Here's the drawing with two shaded views (mm, measured from the low corner). I have some questions. Coordinates: 2 decimals unless noted, no trailing zeros. Write each loop counter-clockwise with the first axis right and the second up, starting at its lowest first coordinate (ties: lowest second). Pieces come first, ordered by that corner, then holes. Notation, with made-up numbers: M 71.25,67.5 L 113.25,67.5 A24 ccw 113.25,99.5 Z; hole C -15.5,-20 d1. An arc over 180 degrees is marked long. Use one line per item in the form item = value. Start each with the question number.
1. I want a section at A-A, the plane y = 2.25. List the corners of the cut face in (x, z) for me.
2. I want a section at B-B, the plane y = 5.25. List the corners of the cut face in (x, z) for me.
3. I'm going to push a flat-ended pin straight in: pin 1 Ø2 at (x, y) = (2, 1.5) entering from +Z. Where does the tip first touch, or does it pass through?
4. Thinking about a two-plate mould opening in X: for the marked faces 1, 2 and 3, which applies, released by +X, released by -X, zero draft, split by the parting line, or undercut?
5. Please list where these lines run through material, in increasing order: line 1 along X through (y, z) = (4.5, 2.05); line 2 along Z through (x, y) = (1.5, 4.5); line 3 along Y through (x, z) = (2.8, 1.5). Write a range as [from, to].
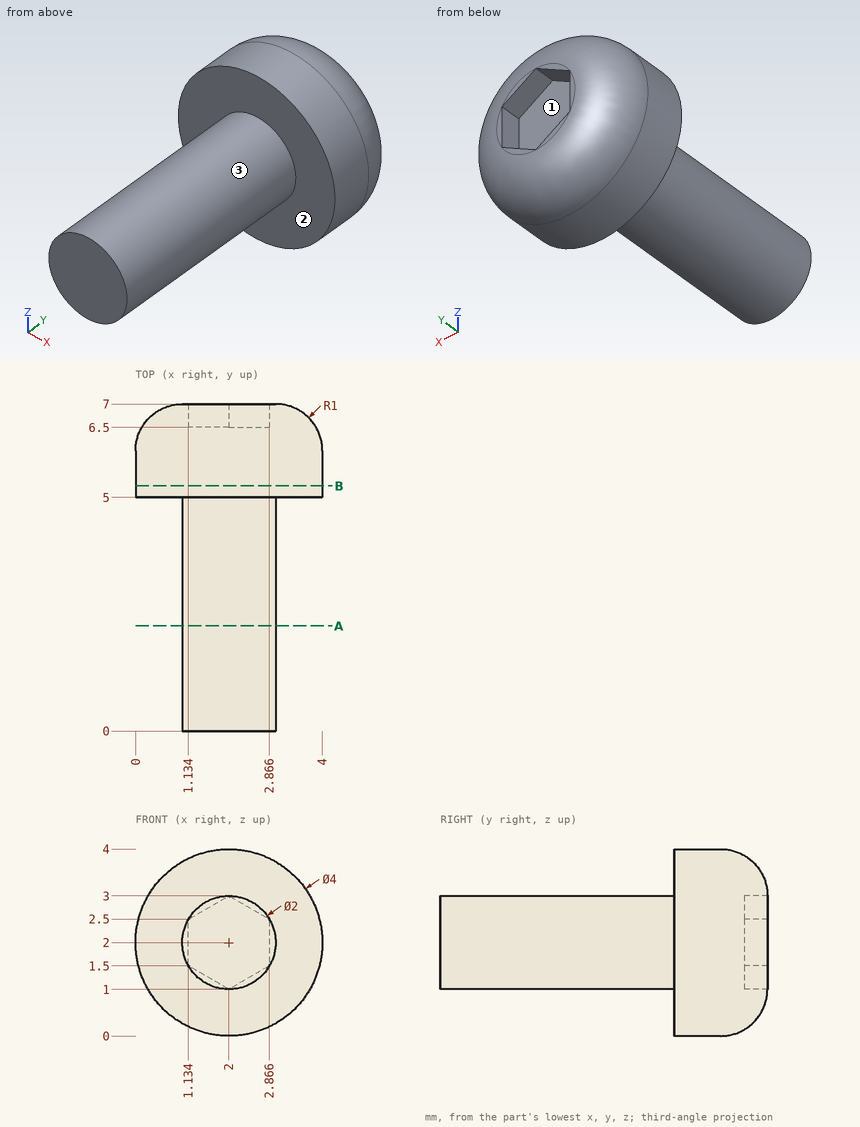
Answer list:
q1.outline = C 2,2 d2
q2.outline = C 2,2 d4
q3.pin_1 = 3
q4.face_1 = undercut
q4.face_2 = zero draft
q4.face_3 = split by the parting line
q5.line_1 = [1, 3]
q5.line_2 = [1.13, 2.87]
q5.line_3 = [0, 6.5]
